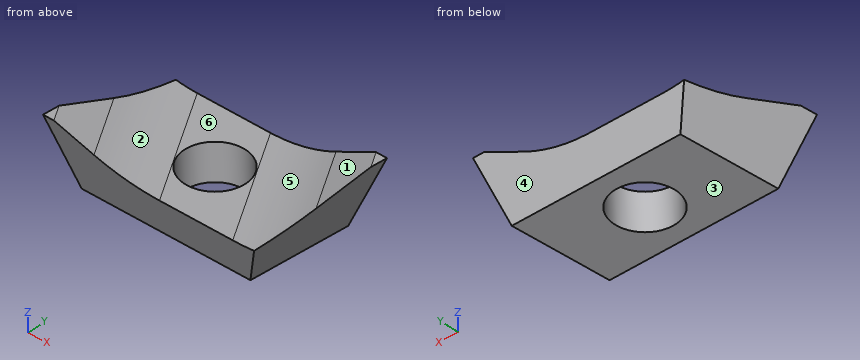
```python
from build123d import *

# Parameters (mm, degrees)
F0_W      = 12
F0_H      = 7
F1_DEPTH  = 3.5
F3_DEPTH  = 7.001
F5_DEPTH  = 12.001
F12_DEPTH = 12.5
F13_R     = 1.65
F14_DEPTH = 2.0010001
F15_R     = 7


with BuildPart() as f1:
    # F0 (on Top) → F1 (new body)
    with BuildSketch(Plane.XY):
        with Locations((6, 3.5)):
            Rectangle(F0_W, F0_H)
    extrude(amount=F1_DEPTH)

    # F2 (on face) → F3 (cut, through all)
    with BuildSketch(Plane.XZ):
        Polygon((1.2738958199, 0), (0, 3.5), (0, 0), align=None)
        Polygon((12, 0), (12, 3.5), (10.7261041801, 0), align=None)
    extrude(amount=-F3_DEPTH, mode=Mode.SUBTRACT)

    # F4 (on Right) → F5 (cut, through all)
    with BuildSketch(Plane.YZ):
        Polygon((0.87264801, 0), (0, 3.5), (0, 0), align=None)
        Polygon((6.12735199, 0), (7, 0), (7, 3.5), align=None)
    extrude(amount=F5_DEPTH, mode=Mode.SUBTRACT)

    # F6 (on face) → F8 section 0
    with BuildSketch(Plane.XY.offset(3.5)):
        Polygon((0, 7), (0, 0), (0.6124206447, 7), align=None)
    # F7 (on face) → F8 section 1
    with BuildSketch(Plane(origin=(0, 0, 0), x_dir=(1, 0, 0), z_dir=(0, 0, -1))):
        Polygon((1.2738958199, -0.87264801), (1.2738958199, -6.12735199), (1.7336228484, -6.12735199), align=None)
    loft(mode=Mode.SUBTRACT)

    # F6 (on face) → F9 section 0
    with BuildSketch(Plane.XY.offset(3.5)):
        Polygon((12, 7), (11.3875793553, 0), (12, 0), align=None)
    # F7 (on face) → F9 section 1
    with BuildSketch(Plane(origin=(0, 0, 0), x_dir=(1, 0, 0), z_dir=(0, 0, -1))):
        Polygon((10.7261041801, -0.87264801), (10.2663771516, -0.87264801), (10.7261041801, -6.12735199), align=None)
    loft(mode=Mode.SUBTRACT)

    # F11 (on 3pt) → F12 (cut, symmetric)
    with BuildSketch(Plane(origin=(0, 0, 0), x_dir=(0.8637789009, 0.5038710255, 0), z_dir=(0.5038710255, -0.8637789009, 0))):
        Polygon((9.8363507794, 3.5), (0.5, 3.5), (3.7, 2), (6.9462219947, 2), (10.1924439894, 2), (13.3924439894, 3.5), align=None)
    extrude(amount=F12_DEPTH, both=True, mode=Mode.SUBTRACT)

    # F13 (on face) → F14 (cut, through all)
    with BuildSketch(Plane.XY.offset(2)):
        with Locations((6, 3.5)):
            Circle(F13_R)
    extrude(amount=-F14_DEPTH, mode=Mode.SUBTRACT)

    # F15
    f15_edges = [f1.edges().sort_by_distance(p)[0] for p in [
        (2.535148, 2.997181, 2),
        (9.464852, 4.002819, 2),
    ]]
    fillet(f15_edges, radius=F15_R)


solid = f1.part
```
Source: CAD feature listing. Evaluate the final solid. Frame: model axes, mm. Face numbers are marked on the shaded views. A direction names the side the tool comes from. Coordinates: 2 decimals unless noted, no trailing zeros. Loops run counter-clockwise (first coordinate to the right, second up) from the corner with the lowest first, then second, coordinate; pieces in that order, holes last. Notation, with made-up numbers: (76, 57) - (98, 57) arc R18 cw to (98, 76) - close; hole circle Ø10 at (79, 55.25). An arc over 180 degrees is marked (long way). Answer as CSV lines item,"result".
1. Mould query, pull axis X, two halves, no side actions, for the marked faces 1, 2 and 3. Classes: released by +X, released by -X, zero draft, split by the parting line, or undercut.
Established:
face 1,"released by -X"
face 2,"undercut"
face 3,"zero draft"
2. Contact query for flat-ended pins moving along their axis: pin 1 (2 mm diameter, centred on y = 5, z = 0.5, fed in from -X); pin 2 (1 mm diameter, centred on x = 10, y = 3.5, fed in from +Z); pin 3 (2 mm diameter, centred on x = 8.5, y = 6, fed in from +Z). Output: stop coordinate, or through.
Established:
pin 1,"stops at x = 1.11"
pin 2,"stops at z = 2.38"
pin 3,"stops at z = 2.56"
3. Reachability of the marked faces 4, 5 and 6 from +Z, -Z, +X, -X, +Y, -Y: full face, straight path, thin tool, end or side. Return the list, or none.
Established:
face 4,"-Z, +X, -X, +Y"
face 5,"+Z, -Y"
face 6,"+Z"
4. Ray query, line 1 (Y direction, x = 6, z = 1); line 2 (X direction, y = 3.25, z = 0.8); line 3 (Y direction, x = 6.75, z = 1). Return the intervals inside material, ascending.
Established:
line 1,"y = 0.62 to 1.85, 5.15 to 6.38"
line 2,"x = 1.21 to 4.37, 7.63 to 10.75"
line 3,"y = 0.62 to 2.03, 4.97 to 6.38"
5. Section A-A (x = 6). Return loops of the section in (y, z).
Established:
outline,"(0.37, 2) - (0.87, 0) - (1.85, 0) - (1.85, 2) - close; (5.15, 0) - (6.13, 0) - (6.63, 2) - (5.15, 2) - close"
